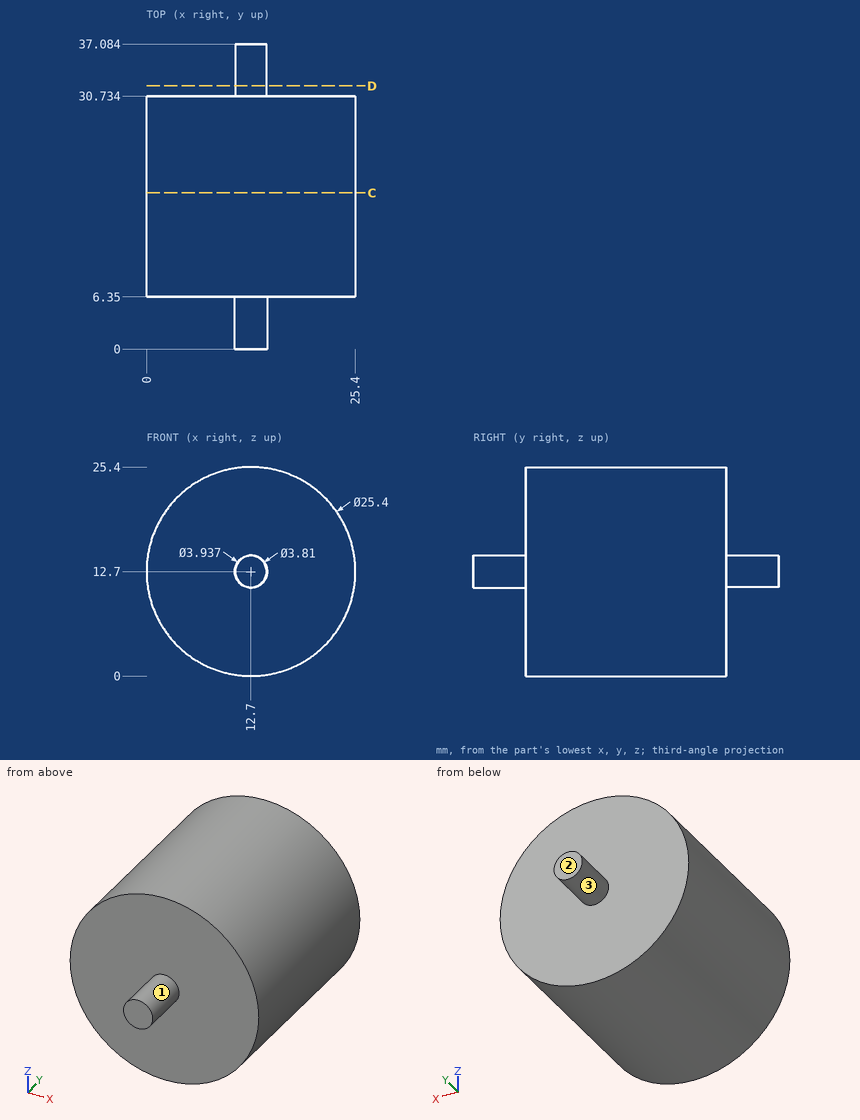
Input: dimensioned drawing with shaded views. Units: mm. Origin: part minimum x, y, z. A direction names the side the tool comes from. Round coordinates to 2 decimals unless told otherwise and drop trailing zeros. Order: outer loops, then holes, each group sorted by start corner. A loop starts at its lowest first (then second) coordinate and runs counter-clockwise, first axis right, second up.
1. Pin query (flat end, axial travel): P1, Ø6, axis at x = 17.5, y = 17, coming from the -Z side; P2, Ø10, axis at x = 18, y = 15, coming from the -Z side; P3, Ø7.5, axis at x = 17.5, z = 9.5, coming from the -Y side. Return the tip coordinate at first contact, or that it passes through.
The answers:
P1: stops at z = 0.13
P2: stops at z = 0
P3: stops at y = 6.35
2. Cut plane D-D, the plane y = 32. Output: boundary loops of the cut face in (x, z) (3 decimals).
The answers:
outline: circle Ø3.81 at (12.7, 12.7)
3. Set-up query: the marked faces 1, 2 and 3. Return all of +Z, -Z, +X, -X, +Y, -Y with unobstructed straight access to the full face (end or side cutting, diameter ignored); none if empty.
The answers:
face 1: -Y
face 2: +Z, -Z, +X, -X, +Y
face 3: +Y
4. Cut plane C-C, the plane y = 19. Output: boundary loops of the cut face in (x, z), then the cut area to 3 significant figures.
The answers:
outline: circle Ø25.4 at (12.7, 12.7)
area: 507 mm2
5. Material intervals for line 1 (Y direction, x = 3, z = 11); line 2 (Z direction, x = 15.25, y = 28); line 3 (Z direction, x = 2, y = 20), sorted ascending.
The answers:
line 1: y = 6.35 to 30.73
line 2: z = 0.26 to 25.14
line 3: z = 5.86 to 19.54
